```python
from build123d import *

# Parameters (mm, degrees)
CROQUIS1_R              = 100
SALIENTE_EXTRUIR1_DEPTH = 3
CROQUIS3_R              = 110
CORTAR_EXTRUIR1_DEPTH   = 3
REDONDEO1_R             = 10
CORTAR_EXTRUIR3_DEPTH   = 10
CROQUIS10_R             = 1.5
CORTAR_EXTRUIR4_DEPTH   = 142.453172607
CROQUIS12_R             = 1.5
CORTAR_EXTRUIR6_DEPTH   = 142.453172607
CROQUIS13_R             = 2
CORTAR_EXTRUIR7_DEPTH   = 142.453172607
CROQUIS15_W             = 32
CROQUIS15_H             = 35
CORTAR_EXTRUIR8_DEPTH   = 142.453172607
REDONDEO2_R             = 3
CROQUIS16_R             = 1.5
CORTAR_EXTRUIR9_DEPTH   = 142.453172607
CROQUIS17_W             = 20
CROQUIS17_H             = 55
CORTAR_EXTRUIR10_DEPTH  = 142.453172607
REDONDEO3_R             = 10


with BuildPart() as part:
    # Croquis1 → Saliente-Extruir1 (new body)
    with BuildSketch(Plane.XY):
        Circle(CROQUIS1_R)
    extrude(amount=SALIENTE_EXTRUIR1_DEPTH)

    # Croquis3 → Cortar-Extruir1 (cut)
    with BuildSketch(Plane.XY.offset(3)):
        with Locations((190, 0)):
            Circle(CROQUIS3_R)
    extrude(amount=-CORTAR_EXTRUIR1_DEPTH, mode=Mode.SUBTRACT)

    # Redondeo1
    redondeo1_edges = [part.edges().sort_by_distance(p)[0] for p in [
        (89.473684211, -44.659375654, 1.5),
        (89.473684211, 44.659375654, 1.5),
    ]]
    fillet(redondeo1_edges, radius=REDONDEO1_R)

    # Croquis7 → Cortar-Extruir3 (cut)
    with BuildSketch(Plane.XY.offset(3)):
        Polygon((-71.939339828, -40.119534675), (-40.119534675, -71.939339828), (-57.797204204, -89.617009358), (-89.617009358, -57.797204204), align=None)
        Polygon((-40.119534675, 71.939339828), (-71.939339828, 40.119534675), (-89.617009358, 57.797204204), (-57.797204204, 89.617009358), align=None)
        Polygon((71.939339828, 40.119534675), (40.119534675, 71.939339828), (57.797204204, 89.617009358), (89.617009358, 57.797204204), align=None)
        Polygon((40.119534675, -71.939339828), (71.939339828, -40.119534675), (89.617009358, -57.797204204), (57.797204204, -89.617009358), align=None)
    extrude(amount=-CORTAR_EXTRUIR3_DEPTH, mode=Mode.SUBTRACT)

    # Croquis10 → Cortar-Extruir4 (cut, through all)
    with BuildSketch(Plane.XY.offset(3)):
        with Locations((-20, 8.5)):
            Circle(CROQUIS10_R)
    extrude(amount=-CORTAR_EXTRUIR4_DEPTH, mode=Mode.SUBTRACT)

    # Croquis12 → Cortar-Extruir6 (cut, through all)
    with BuildSketch(Plane(origin=(0, 0, 0), x_dir=(-1, 0, 0), z_dir=(0, 0, -1))):
        with Locations((-71, 11)):
            Circle(CROQUIS12_R)
        with Locations((-71, -11)):
            Circle(CROQUIS12_R)
        with Locations((-60, 11)):
            Circle(CROQUIS12_R)
        with Locations((-60, -11)):
            Circle(CROQUIS12_R)
    extrude(amount=-CORTAR_EXTRUIR6_DEPTH, mode=Mode.SUBTRACT)

    # Croquis13 → Cortar-Extruir7 (cut, through all)
    with BuildSketch(Plane(origin=(0, 0, 0), x_dir=(-1, 0, 0), z_dir=(0, 0, -1))):
        with Locations((0, 92)):
            Circle(CROQUIS13_R)
        with Locations((0, -92)):
            Circle(CROQUIS13_R)
        with Locations((70.711068531, 30)):
            Circle(CROQUIS13_R)
        with Locations((70.711643931, -30)):
            Circle(CROQUIS13_R)
        with Locations((-60, 20)):
            Circle(CROQUIS13_R)
        with Locations((-60, -20)):
            Circle(CROQUIS13_R)
    extrude(amount=-CORTAR_EXTRUIR7_DEPTH, mode=Mode.SUBTRACT)

    # Croquis15 → Cortar-Extruir8 (cut, through all)
    with BuildSketch(Plane(origin=(0, 0, 0), x_dir=(-1, 0, 0), z_dir=(0, 0, -1))):
        Polygon((18.226497308, 55), (-34.226497308, 55), (-28.452994616, 45), (-34.226497308, 35), (18.226497308, 35), (12.452994616, 45), align=None)
        Polygon((-34.226497308, 55), (-40, 55), (-40, 35), (-34.226497308, 35), (-28.452994616, 45), align=None)
        Polygon((-40, 35), (-40, 55), (-45.773502692, 55), (-51.547005384, 45), (-45.773502692, 35), align=None)
        Polygon((29.773502692, 55), (24, 55), (24, 35), (29.773502692, 35), (35.547005384, 45), align=None)
        Polygon((24, 55), (18.226497308, 55), (12.452994616, 45), (18.226497308, 35), (24, 35), align=None)
        Polygon((12.452994616, -45), (18.226497308, -35), (-34.226497308, -35), (-28.452994616, -45), (-34.226497308, -55), (18.226497308, -55), align=None)
        Polygon((24, -55), (24, -35), (18.226497308, -35), (12.452994616, -45), (18.226497308, -55), align=None)
        Polygon((35.547005384, -45), (29.773502692, -35), (24, -35), (24, -55), (29.773502692, -55), align=None)
        Polygon((-28.452994616, -45), (-34.226497308, -35), (-40, -35), (-40, -55), (-34.226497308, -55), align=None)
        Polygon((-40, -55), (-40, -35), (-45.773502692, -35), (-51.547005384, -45), (-45.773502692, -55), align=None)
        with Locations((48, 0)):
            Rectangle(CROQUIS15_W, CROQUIS15_H)
    extrude(amount=-CORTAR_EXTRUIR8_DEPTH, mode=Mode.SUBTRACT)

    # Redondeo2
    redondeo2_edges = [part.edges().sort_by_distance(p)[0] for p in [
        (-64, 17.5, 1.5),
        (-32, 17.5, 1.5),
        (-32, -17.5, 1.5),
        (-64, -17.5, 1.5),
    ]]
    fillet(redondeo2_edges, radius=REDONDEO2_R)

    # Croquis16 → Cortar-Extruir9 (cut, through all)
    with BuildSketch(Plane(origin=(0, 0, 0), x_dir=(-1, 0, 0), z_dir=(0, 0, -1))):
        with Locations((-19.5, 65)):
            Circle(CROQUIS16_R)
        with Locations((19.5, 65)):
            Circle(CROQUIS16_R)
        with Locations(Location((19.5, -65, 0), (0, 0, 180))):
            Circle(CROQUIS16_R)
        with Locations(Location((-19.5, -65, 0), (0, 0, 180))):
            Circle(CROQUIS16_R)
        with Locations((36, 35)):
            Circle(CROQUIS16_R)
        with Locations((36, -35)):
            Circle(CROQUIS16_R)
        with Locations((60, -35)):
            Circle(CROQUIS16_R)
        with Locations((60, 35)):
            Circle(CROQUIS16_R)
        with Locations((92, 19.5)):
            Circle(CROQUIS16_R)
        with Locations((92, -19.5)):
            Circle(CROQUIS16_R)
    extrude(amount=-CORTAR_EXTRUIR9_DEPTH, mode=Mode.SUBTRACT)

    # Croquis17 → Cortar-Extruir10 (cut, through all)
    with BuildSketch(Plane(origin=(0, 0, 0), x_dir=(-1, 0, 0), z_dir=(0, 0, -1))):
        with Locations((-26, 0)):
            Rectangle(CROQUIS17_W, CROQUIS17_H)
    extrude(amount=-CORTAR_EXTRUIR10_DEPTH, mode=Mode.SUBTRACT)

    # Redondeo3
    redondeo3_edges = [part.edges().sort_by_distance(p)[0] for p in [
        (16, -27.5, 1.5),
        (36, -27.5, 1.5),
        (16, 27.5, 1.5),
        (36, 27.5, 1.5),
    ]]
    fillet(redondeo3_edges, radius=REDONDEO3_R - 0.0001)  # a hair under: the kernel refuses the full size


solid = part.part
```
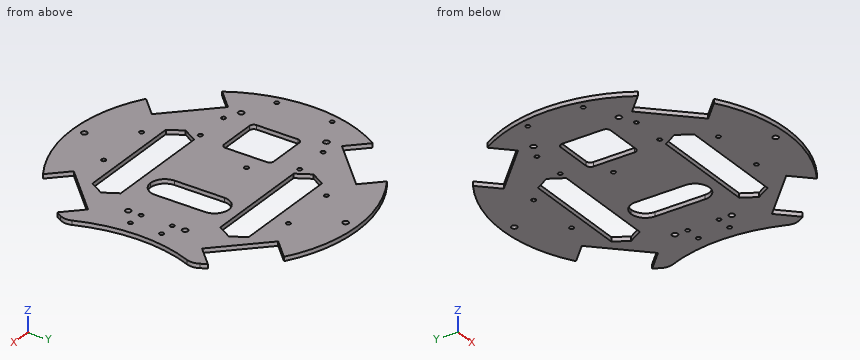
Input: part model. Units: mm. Frame: model coordinates. Coordinates: 2 decimals unless noted, no trailing zeros. Write each loop counter-clockwise with the first axis right and the second up, starting at its lowest first coordinate (ties: lowest second). Pieces come first, ordered by that corner, then holes. Notation, with made-up numbers: (63, 68.5) -> (102, 68.5) arc R35 cw to (102, 106.5) -> close; hole circle Ø3 at (36.25, 21.5). An arc over 180 degrees is marked (long way). Answer as a JSON object with one key per item and string values.
1. Section A-A on x = 29.5. Return the cut outline in (y, z).
Result set:
{"outline": "(-95.55, 0) -> (-55, 0) -> (-55, 3) -> (-95.55, 3) -> close; (-35, 0) -> (-26.87, 0) -> (-26.87, 3) -> (-35, 3) -> close; (26.87, 0) -> (35, 0) -> (35, 3) -> (26.87, 3) -> close; (55, 0) -> (95.55, 0) -> (95.55, 3) -> (55, 3) -> close"}
2. Material intervals for line 1 (X direction, y = 1, z = 0.95) (3 decimals); line 2 (Y direction, x = -49, z = 1.95); line 3 (Y direction, x = -22.5, z = 2.3), sorted ascending. Write a range as from..to.
Result set:
{"line 1": "x = -99.995..-64, -32..16, 36..80.005", "line 2": "y = -87.17..-80.82, -63.06..-17.5, 17.5..63.06, 80.82..87.17", "line 3": "y = -97.44..-55, -35..35, 55..97.44"}
3. Section D-D on y = -78. Return the cut outline in (x, z), then the cut area to 3 significant figures.
Result set:
{"outline": "(-46.18, 0) -> (46.18, 0) -> (46.18, 3) -> (-46.18, 3) -> close", "area": "277 mm2"}
4. Section C-C on z = 0.8. Count the separate pieces of the cut face and the enclosed holes in it, then the cut area to 3 significant figures.
Result set:
{"separate pieces": "1", "enclosed holes": "25", "area": "21,100 mm2"}
5. First-contact query: P1, Ø0.9, axis at x = 18, z = 2, coming from the -Y side; P2, Ø1.5, axis at x = 49.5, z = 2, coming from the -Y side. Flat tips, straight axial feed; report the tip coordinate or a pass-through.
Result set:
{"P1": "stops at y = -98.45", "P2": "stops at y = -87.31"}
6. Section B-B on x = -14.5. Return the cut outline in (y, z), then the cut area to 3 significant figures.
Result set:
{"outline": "(-98.94, 0) -> (-55, 0) -> (-55, 3) -> (-98.94, 3) -> close; (-35, 0) -> (35, 0) -> (35, 3) -> (-35, 3) -> close; (55, 0) -> (98.94, 0) -> (98.94, 3) -> (55, 3) -> close", "area": "474 mm2"}
